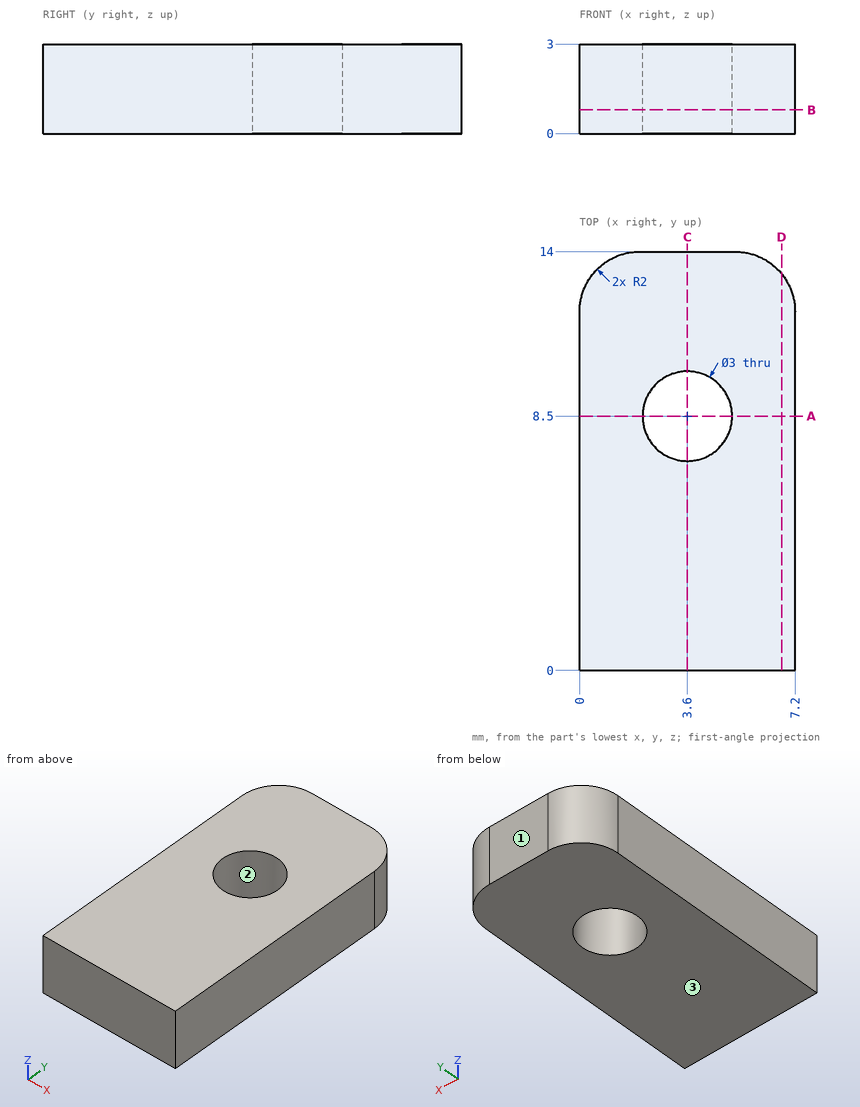
Answer from the drawing. Dimensions are ordinates in mm from the lowest x, y and z of the part. Coordinates: 2 decimals unless noted, no trailing zeros. Loops run counter-clockwise (first coordinate to the right, second up) from the corner with the lowest first, then second, coordinate; pieces in that order, holes last.
1) Section B-B (z = 0.8) is taken. Give the vertices of the cut face in (x, y), plus the area to 3 significant figures.
Results:
outline: (0, 0) - (7.2, 0) - (7.2, 12) arc R2 ccw to (5.2, 14) - (2, 14) arc R2 ccw to (0, 12) - close; hole circle Ø3 at (3.6, 8.5)
area: 92.0 mm2
2) For a pull along Y with two mould halves and no side action, classify the marked faces 1, 2 and 3 as +Y half, -Y half, draft (parallel to the pull), parting line (faces both ways), or undercut.
Results:
face 1: +Y half
face 2: undercut
face 3: draft
3) Section D-D (x = 6.75) is taken. Give the vertices of the cut face in (y, z).
Results:
outline: (0, 0) - (13.26, 0) - (13.26, 3) - (0, 3) - close
4) Section A-A (y = 8.5) is taken. Give the vertices of the cut face in (x, z).
Results:
outline: (0, 0) - (2.1, 0) - (2.1, 3) - (0, 3) - close; (5.1, 0) - (7.2, 0) - (7.2, 3) - (5.1, 3) - close
5) Consider probe 1 along Y at (x, z) = (3.6, 1.4); probe 2 along Y at (x, z) = (4.5, 0.8); probe 3 along Y at (x, z) = (0.75, 1.7). Determine where each line is inside the solid, lowest interval first.
Results:
probe 1: y = 0 to 7, 10 to 14
probe 2: y = 0 to 7.3, 9.7 to 14
probe 3: y = 0 to 13.56
6) Section C-C (x = 3.6) is taken. Give the vertices of the cut face in (y, z).
Results:
outline: (0, 0) - (7, 0) - (7, 3) - (0, 3) - close; (10, 0) - (14, 0) - (14, 3) - (10, 3) - close
